from build123d import *

# Parameters (mm, degrees)
SKETCH1_W           = 10
SKETCH1_H           = 8
BOSS_EXTRUDE1_DEPTH = 2
SKETCH2_W           = 10
SKETCH2_H           = 2
BOSS_EXTRUDE2_DEPTH = 8
SKETCH3_R           = 1.5
CUT_EXTRUDE1_DEPTH  = 10.848857802
SKETCH4_R           = 1.5
CUT_EXTRUDE2_DEPTH  = 13.369316877
FILLET1_R           = 0.5


with BuildPart() as part:
    # Sketch1 → Boss-Extrude1 (new body)
    with BuildSketch(Plane(origin=(0, 0, 0), x_dir=(1, 0, 0), z_dir=(0, 1, 0))):
        Rectangle(SKETCH1_W, SKETCH1_H)
    extrude(amount=BOSS_EXTRUDE1_DEPTH)

    # Sketch2 → Boss-Extrude2 (add)
    with BuildSketch(Plane(origin=(0, 0, 0), x_dir=(1, 0, 0), z_dir=(0, 1, 0))):
        with Locations((0, 5)):
            Rectangle(SKETCH2_W, SKETCH2_H)
    extrude(amount=BOSS_EXTRUDE2_DEPTH)

    # Sketch3 → Cut-Extrude1 (cut, through all)
    with BuildSketch(Plane(origin=(0, 2, 0), x_dir=(1, 0, 0), z_dir=(0, 1, 0))):
        with Locations(Location((0, -1, 0), (0, 0, 270))):
            Circle(SKETCH3_R)
    extrude(amount=-CUT_EXTRUDE1_DEPTH, mode=Mode.SUBTRACT)

    # Sketch4 → Cut-Extrude2 (cut, through all)
    with BuildSketch(Plane.XY.offset(-4)):
        with Locations((0, 5)):
            Circle(SKETCH4_R)
    extrude(amount=-CUT_EXTRUDE2_DEPTH, mode=Mode.SUBTRACT)

    # Fillet1
    fillet1_edges = [part.edges().sort_by_distance(p)[0] for p in [
        (-5, 2, 0),
        (5, 5, -4),
        (0, 0, -6),
        (5, 4, -6),
        (-5, 4, -6),
        (-5, 5, -4),
        (5, 8, -5),
        (0, 8, -6),
        (0, 2, 4),
        (-5, 8, -5),
        (0, 8, -4),
        (5, 2, 0),
        (0, 0, 4),
        (-5, 0, -1),
        (5, 0, -1),
        (5, 1, 4),
        (-5, 1, 4),
        (0, 2, -4),
    ]]
    fillet(fillet1_edges, radius=FILLET1_R)


solid = part.part
Input: part model. Units: mm. Frame: model coordinates. A direction names the side the tool comes from. Give positions to 0.01 mm unless a question says otherwise; leave off trailing zeros. Loops run counter-clockwise (first coordinate to the right, second up) from the corner with the lowest first, then second, coordinate; pieces in that order, holes last. Notation, with made-up numbers: (13, -29) - (24, -29) arc R10 cw to (24, -22) - close; hole circle Ø7 at (73, 86). An arc over 180 degrees is marked (long way). Use CSV: the item, a comma, the result in double quotes. Start each with the question number.
Item 1: Section D-D on y = 5. Return loops of the section in (x, z), then the cut area to 3 significant figures.
Item 2: Reachability of faces 4 (the flat face through (0, 1, 4)), 5 (the flat face through (0, 2, -1)) from +Z, -Z, +X, -X, +Y, -Y: full face, straight path, thin tool, end or side. Return the list, or none.
Item 3: Section A-A on y = 1.25. Return loops of the section in (x, z), then the cut area to 3 significant figures.
Item 4: Section B-B on z = -4.75. Return loops of the section in (x, y), then the cut area to 3 significant figures.
Item 5: Section C-C on x = 0. Return loops of the section in (y, z), then the cut area to 3 significant figures.
Item 6: Contact query for flat-ended pins moving along their axis: P1, Ø1.5, axis at x = 1, y = 5, coming from the +Z side; P2, Ø3.5, axis at x = 0, z = 1, coming from the +Y side; P3, Ø5.5, axis at x = -2, z = -1.5, coming from the +Y side; P4, Ø2.5, axis at x = 0, y = 5, coming from the +Z side. Output: stop coordinate, or through.
Item 7: Mould query, pull axis X, two halves, no side actions, for faces 1 (the flat face through (0, 7, -4)), 2 (the flat face through (-5, 1, -3)), 3 (the cylindrical face through (-1.5, 5.07, -4.99)). Classes: pulls with the +X half, pulls with the -X half, needs draft (parallel to the pull), parting line crosses it, or undercut.
Item 8: Line query: line 1 (Y direction, x = 0, z = -4.6); line 2 (Y direction, x = -3, z = -3.5); line 3 (Z direction, x = 0.75, y = 3). Output: solid intervals per line, ascending.
Ans:
1,outline,"(-5, -5.5) arc R0.5 ccw to (-4.5, -6) - (-1.5, -6) - (-1.5, -4) - (-4.5, -4) arc R0.5 ccw to (-5, -4.5) - close; (1.5, -6) - (4.5, -6) arc R0.5 ccw to (5, -5.5) - (5, -4.5) arc R0.5 ccw to (4.5, -4) - (1.5, -4) - close"
1,area,"13.8 mm2"
2,face 4,"+Z, +X, -X, +Y, -Y"
2,face 5,"+Z, +X, -X, +Y"
3,outline,"(-5, -5.5) arc R0.5 ccw to (-4.5, -6) - (4.5, -6) arc R0.5 ccw to (5, -5.5) - (5, 3.5) arc R0.5 ccw to (4.5, 4) - (-4.5, 4) arc R0.5 ccw to (-5, 3.5) - close; hole circle Ø3 at (0, 1)"
3,area,"92.7 mm2"
4,outline,"(-5, 0.5) arc R0.5 ccw to (-4.5, 0) - (4.5, 0) arc R0.5 ccw to (5, 0.5) - (5, 7.5) arc R0.5 ccw to (4.5, 8) - (-4.5, 8) arc R0.5 ccw to (-5, 7.5) - close; hole circle Ø3 at (0, 5)"
4,area,"72.7 mm2"
5,outline,"(0, -5.5) arc R0.5 ccw to (0.5, -6) - (3.5, -6) - (3.5, -4) - (2.5, -4) arc R0.5 cw to (2, -3.5) - (2, -0.5) - (0, -0.5) - close; (0, 2.5) - (2, 2.5) - (2, 3.5) arc R0.5 ccw to (1.5, 4) - (0.5, 4) arc R0.5 ccw to (0, 3.5) - close; (6.5, -6) - (7.5, -6) arc R0.5 ccw to (8, -5.5) - (8, -4.5) arc R0.5 ccw to (7.5, -4) - (6.5, -4) - close"
5,area,"19.8 mm2"
6,P1,"stops at z = -4"
6,P2,"stops at y = 2"
6,P3,"stops at y = 7.93"
6,P4,"passes through"
7,face 1,"needs draft"
7,face 2,"pulls with the -X half"
7,face 3,"undercut"
8,line 1,"y = 0 to 3.5, 6.5 to 8"
8,line 2,"y = 0 to 2"
8,line 3,"z = -6 to -4"
